Autodesk Inventor part; units mm, degrees
ref_plane "YZ Plane" through (0, 0, 0) normal (1, 0, 0) x (0, 1, 0)
ref_plane "XZ Plane" through (0, 0, 0) normal (0, 1, 0) x (-1, 0, 0)
ref_plane "XY Plane" through (0, 0, 0) normal (0, 0, 1) x (1, 0, 0)
sketch "Sketch1" plane through (0, 0, 0) normal (0, 0, 1) x (1, 0, 0)
  line L0 (-12.1708, 16.0073) -> (13.2292, 16.0073)
  line L1 (13.2292, 16.0073) -> (13.2292, -34.7927)
  line L2 (13.2292, -34.7927) -> (-12.1708, -34.7927)
  line L3 (-12.1708, -34.7927) -> (-12.1708, 16.0073)
  line L4 (11.9592, 14.7373) -> (-10.9008, 14.7373)
  line L5 (-10.9008, 14.7373) -> (-10.9008, -33.5227)
  line L6 (-10.9008, -33.5227) -> (11.9592, -33.5227)
  line L7 (11.9592, -33.5227) -> (11.9592, 14.7373)
  point P0 (0, 0)
  dimension "d0" = 25.4
  dimension "d1" = 50.8
  dimension "d2" = 1.27
extrude "Extrusion1" add sketch "Sketch1" along normal blind 203.2
sketch "Sketch2" plane through (-12.1708, 16.0073, 0) normal (0, 1, 0) x (1, 0, 0)
  circle A0 centre (12.7, -12.7) radius 1.7272
  line L0 (25.4, 0) -> (0, 0)
  line L1 (0, 0) -> (0, -203.2)
  point P0 (12.1708, 0)
  dimension "d5" = 3.4544
  dimension "d6" = 12.7
  dimension "d7" = 12.7
extrude "Extrusion2" cut sketch "Sketch2" against normal through all
pattern_linear "Rectangular Pattern1" count 20 spacing 25.4 along (0, 0, 1) of "Extrusion2"
equation "\"d3\" = d13"
equation "\"d10\" = d14"
equation "\"d13\" = 203.2"
equation "\"d14\" = d13"
properties part number "VersaFrame (Gripper-StationaryLong)"
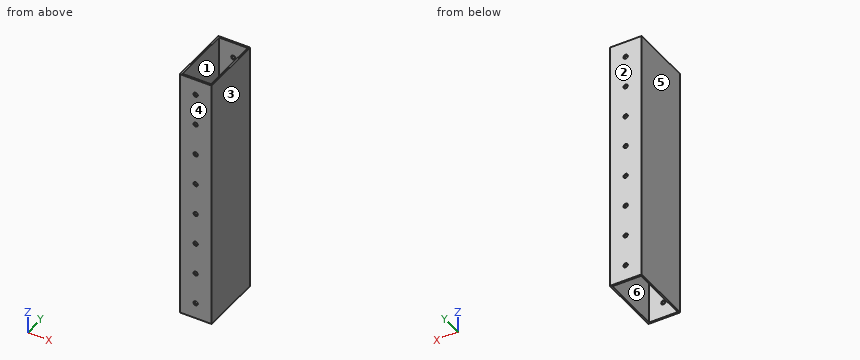
Build history of the part. All positions in model axes, mm. Face numbers are marked on the shaded views. A direction names the side the tool comes from. Give positions to 0.01 mm unless a question says otherwise; leave off trailing zeros. Loops run counter-clockwise (first coordinate to the right, second up) from the corner with the lowest first, then second, coordinate; pieces in that order, holes last. Notation, with made-up numbers: (2, 87.25) -> (7, 87.25) arc R16 cw to (7, 101.25) -> close; hole circle Ø4 at (-22, 43). An arc over 180 degrees is marked (long way). Answer in a Markdown table with one row per item.
Item 1: Probe line 1 along X through (y, z) = (-9, 146); line 2 along Y through (x, z) = (-4, 113); line 3 along X through (y, z) = (-34, 165). List the from-to ranges inside material, lowest first. Write a range as [from, to].
Findings below:
| item | result |
|---|---|
| line 1 | x = [-12.17, -10.9], [11.96, 13.23] |
| line 2 | y = [-34.79, -33.52], [14.74, 16.01] |
| line 3 | x = [-12.17, -1.2], [2.25, 13.23] |
Item 2: Tool access for the marked faces 5 and 6: list every direction of +Z, -Z, +X, -X, +Y, -Y with a clear straight run to the whole face (end or side of a thin tool).
Findings below:
| item | result |
|---|---|
| face 5 | +Z, -Z, -X, +Y, -Y |
| face 6 | +Z, -Z |
Item 3: Mould opens along Y. For the marked faces 1, 2, 3 and 4 say: pulls with the +Y half, pulls with the -Y half, needs draft (parallel to the pull), parting line crosses it, or undercut.
Findings below:
| item | result |
|---|---|
| face 1 | undercut |
| face 2 | pulls with the +Y half |
| face 3 | needs draft |
| face 4 | pulls with the -Y half |
Item 4: Slice it at A-A on x = 6. Write the cut outline in (y, z), plus the area to 3 significant figures.
Findings below:
| item | result |
|---|---|
| outline | (-34.79, 0) -> (-33.52, 0) -> (-33.52, 203.2) -> (-34.79, 203.2) -> close; (14.74, 0) -> (16.01, 0) -> (16.01, 203.2) -> (14.74, 203.2) -> close |
| area | 516 mm² |
Item 5: Slice it at D-D on z = 75.5. Write the cut outline in (x, y).
Findings below:
| item | result |
|---|---|
| outline | (-12.17, -34.79) -> (13.23, -34.79) -> (13.23, 16.01) -> (-12.17, 16.01) -> close; hole (-10.9, -33.52) -> (11.96, -33.52) -> (11.96, 14.74) -> (-10.9, 14.74) -> close |
Item 6: Slice it at C-C on y = -16.5. Write the cut outline in (x, z), plus the area to 3 significant figures.
Findings below:
| item | result |
|---|---|
| outline | (-12.17, 0) -> (-10.9, 0) -> (-10.9, 203.2) -> (-12.17, 203.2) -> close; (11.96, 0) -> (13.23, 0) -> (13.23, 203.2) -> (11.96, 203.2) -> close |
| area | 516 mm² |
Item 7: Slice it at B-B on z = 190.5. Write the cut outline in (x, y).
Findings below:
| item | result |
|---|---|
| outline | (-12.17, -34.79) -> (-1.2, -34.79) -> (-1.2, -33.52) -> (-10.9, -33.52) -> (-10.9, 14.74) -> (-1.2, 14.74) -> (-1.2, 16.01) -> (-12.17, 16.01) -> close; (2.26, -34.79) -> (13.23, -34.79) -> (13.23, 16.01) -> (2.26, 16.01) -> (2.26, 14.74) -> (11.96, 14.74) -> (11.96, -33.52) -> (2.26, -33.52) -> close |
